```python
from build123d import *

# Parameters (mm, degrees)
BOSS_EXTRUDE1_DEPTH              = 12.7
SKETCH2_R                        = 19.0754
CUT_EXTRUDE2_DEPTH               = 214.127417875
F_10_32_TAPPED_HOLE2_AT_2_COUNT  = 2
F_10_32_TAPPED_HOLE2_AT_2_PITCH  = 101.6
F_10_32_TAPPED_HOLE2_AT_3_COUNT  = 2
F_10_32_TAPPED_HOLE2_AT_3_PITCH  = 199.581369562
F_10_32_TAPPED_HOLE2_AT_4_COUNT  = 2
F_10_32_TAPPED_HOLE2_AT_4_PITCH  = 257.571569241
F_10_32_TAPPED_HOLE2_AT_5_COUNT  = 2
F_10_32_TAPPED_HOLE2_AT_5_PITCH  = 260.369359036
F_10_32_TAPPED_HOLE2_AT_6_COUNT  = 2
F_10_32_TAPPED_HOLE2_AT_6_PITCH  = 236.729200842
F_10_32_TAPPED_HOLE2_AT_7_COUNT  = 2
F_10_32_TAPPED_HOLE2_AT_7_PITCH  = 125.046561074
F_10_32_TAPPED_HOLE2_AT_8_COUNT  = 2
F_10_32_TAPPED_HOLE2_AT_8_PITCH  = 191.941079739
F_1_4_28_TAPPED_HOLE1_AT_2_COUNT = 2
F_1_4_28_TAPPED_HOLE1_AT_2_PITCH = 118.029744238
F_1_4_28_TAPPED_HOLE1_AT_3_COUNT = 2
F_1_4_28_TAPPED_HOLE1_AT_3_PITCH = 162.987319215


with BuildPart() as part:
    # Sketch1 → Boss-Extrude1 (new body)
    with BuildSketch(Plane.XY):
        Polygon((-130.175, -168.275), (130.175, -168.275), (130.175, 60.325), (60.325, 130.175), (-60.325, 130.175), (-130.175, 60.325), align=None)
    extrude(amount=BOSS_EXTRUDE1_DEPTH)

    # Sketch2 → Cut-Extrude2 (cut, through all)
    with BuildSketch(Plane.XY):
        with Locations((0, -57.15)):
            Circle(SKETCH2_R)
    extrude(amount=CUT_EXTRUDE2_DEPTH, mode=Mode.SUBTRACT)

    # Sketch5 → #10-32 Tapped Hole2 (revolve, cut)
    with BuildSketch(Plane(origin=(50.8, 115.8875, 0), x_dir=(0, 1, 0), z_dir=(1, 0, 0))):
        Polygon((0, 0), (0, 12.7), (3.048, 12.7), (2.0193, 11.6713), (2.0193, 1.0287), (3.048, 0), align=None)
    f_10_32_tapped_hole2 = revolve(axis=Axis((50.8, 115.8875, -6.35), (0, 0, 1)), mode=Mode.SUBTRACT)

    # #10-32 Tapped Hole2 at 2: #10-32 Tapped Hole2 ×2
    with Locations(*[(-i * F_10_32_TAPPED_HOLE2_AT_2_PITCH, 0, 0) for i in range(1, F_10_32_TAPPED_HOLE2_AT_2_COUNT)]):
        add(f_10_32_tapped_hole2, mode=Mode.SUBTRACT)

    # #10-32 Tapped Hole2 at 3: #10-32 Tapped Hole2 ×2
    with Locations(*[Vector(-0.8511576023985749, -0.5249102169696354, 0) * (i * F_10_32_TAPPED_HOLE2_AT_3_PITCH) for i in range(1, F_10_32_TAPPED_HOLE2_AT_3_COUNT)]):
        add(f_10_32_tapped_hole2, mode=Mode.SUBTRACT)

    # #10-32 Tapped Hole2 at 4: #10-32 Tapped Hole2 ×2
    with Locations(*[Vector(-0.5547001962252293, -0.8320502943378437, 0) * (i * F_10_32_TAPPED_HOLE2_AT_4_PITCH) for i in range(1, F_10_32_TAPPED_HOLE2_AT_4_COUNT)]):
        add(f_10_32_tapped_hole2, mode=Mode.SUBTRACT)

    # #10-32 Tapped Hole2 at 5: #10-32 Tapped Hole2 ×2
    with Locations(*[Vector(-0.26827273477386476, -0.963343002142514, 0) * (i * F_10_32_TAPPED_HOLE2_AT_5_PITCH) for i in range(1, F_10_32_TAPPED_HOLE2_AT_5_COUNT)]):
        add(f_10_32_tapped_hole2, mode=Mode.SUBTRACT)

    # #10-32 Tapped Hole2 at 6: #10-32 Tapped Hole2 ×2
    with Locations(*[Vector(0.04023584739915886, -0.9991902104124478, 0) * (i * F_10_32_TAPPED_HOLE2_AT_6_PITCH) for i in range(1, F_10_32_TAPPED_HOLE2_AT_6_COUNT)]):
        add(f_10_32_tapped_hole2, mode=Mode.SUBTRACT)

    # #10-32 Tapped Hole2 at 7: #10-32 Tapped Hole2 ×2
    with Locations(*[Vector(0.5459982218929023, -0.8377863341507721, 0) * (i * F_10_32_TAPPED_HOLE2_AT_7_PITCH) for i in range(1, F_10_32_TAPPED_HOLE2_AT_7_COUNT)]):
        add(f_10_32_tapped_hole2, mode=Mode.SUBTRACT)

    # #10-32 Tapped Hole2 at 8: #10-32 Tapped Hole2 ×2
    with Locations(*[Vector(0.35570915873202924, -0.9345967014676182, 0) * (i * F_10_32_TAPPED_HOLE2_AT_8_PITCH) for i in range(1, F_10_32_TAPPED_HOLE2_AT_8_COUNT)]):
        add(f_10_32_tapped_hole2, mode=Mode.SUBTRACT)

    # Sketch7 → 1/4-28 Tapped Hole1 (revolve, cut)
    with BuildSketch(Plane(origin=(105.41, -57.15, 0), x_dir=(0, 1, 0), z_dir=(1, 0, 0))):
        Polygon((0, 0), (0, 12.7), (3.81, 12.7), (2.7051, 11.5951), (2.7051, 1.1049), (3.81, 0), align=None)
    f_1_4_28_tapped_hole1 = revolve(axis=Axis((105.41, -57.15, -6.35), (0, 0, 1)), mode=Mode.SUBTRACT)

    # 1/4-28 Tapped Hole1 at 2: 1/4-28 Tapped Hole1 ×2
    with Locations(*[Vector(-0.09683999633944815, 0.9952999623776622, 0) * (i * F_1_4_28_TAPPED_HOLE1_AT_2_PITCH) for i in range(1, F_1_4_28_TAPPED_HOLE1_AT_2_COUNT)]):
        add(f_1_4_28_tapped_hole1, mode=Mode.SUBTRACT)

    # 1/4-28 Tapped Hole1 at 3: 1/4-28 Tapped Hole1 ×2
    with Locations(*[Vector(-0.35453678407740086, 0.9350420678964421, 0) * (i * F_1_4_28_TAPPED_HOLE1_AT_3_PITCH) for i in range(1, F_1_4_28_TAPPED_HOLE1_AT_3_COUNT)]):
        add(f_1_4_28_tapped_hole1, mode=Mode.SUBTRACT)


solid = part.part
```
Input: part model. Units: mm. Frame: model coordinates. Coordinates: 2 decimals unless noted, no trailing zeros. Loops run counter-clockwise (first coordinate to the right, second up) from the corner with the lowest first, then second, coordinate; pieces in that order, holes last. Notation, with made-up numbers: M -25.75,65.5 L 17.25,65.5 A14 ccw 17.25,92.5 Z; hole C 62.25,52.25 d8. An arc over 180 degrees is marked long. Answer in a Markdown table with one row per item.
1. First-contact query: pin 1 (5.5 mm diameter, centred on x = 119.08, y = 11.13, fed in from +Z); pin 2 (1 mm diameter, centred on x = 95, y = -130, fed in from -Z); pin 3 (2.5 mm diameter, centred on x = 50.8, y = 115.89, fed in from +Z); pin 4 (7 mm diameter, centred on x = 47.625, y = 95.25, fed in from -Z). Flat tips, straight axial feed; report the tip coordinate or a pass-through.
Response:
| item | result |
|---|---|
| pin 1 | stops at z = 12.41 |
| pin 2 | stops at z = 0 |
| pin 3 | passes through |
| pin 4 | stops at z = 0.31 |
2. Section A-A, the plane x = 0. Output: boundary loops of the cut face in (y, z) (3 decimals).
Response:
| item | result |
|---|---|
| outline | M -168.275,0 L -76.225,0 L -76.225,12.7 L -168.275,12.7 Z; M -38.075,0 L 130.175,0 L 130.175,12.7 L -38.075,12.7 Z |
3. Material intervals for line 1 (Y direction, x = 47.5, z = 9.5) (3 decimals); line 2 (X direction, y = 12, z = 9.75) (3 decimals); line 3 (Y direction, x = 50.8, z = 9.5) (3 decimals), sorted ascending.
Response:
| item | result |
|---|---|
| line 1 | y = -168.275 to 92.548, 97.952 to 130.175 |
| line 2 | x = -130.175 to -120.895, -117.255 to 117.255, 120.895 to 130.175 |
| line 3 | y = -168.275 to 113.868, 117.907 to 130.175 |
4. Draft query along Y for faces 1 (the flat face through (95.7, 94.8, 6.3)), 2 (the flat face through (-2, -17, 0)), 3 (the cylindrical face through (-4.14, -75.77, 6.26)). Return one class per face: pulls with the +Y half, pulls with the -Y half, needs draft (parallel to the pull), parting line crosses it, or undercut.
Response:
| item | result |
|---|---|
| face 1 | pulls with the +Y half |
| face 2 | needs draft |
| face 3 | undercut |
5. Section D-D, the plane x = -78.5. Output: boundary loops of the cut face in (y, z) (3 decimals), then the cut area to 3 significant figures.
Response:
| item | result |
|---|---|
| outline | M -168.275,0 L 112,0 L 112,12.7 L -168.275,12.7 Z |
| area | 3,560 mm2 |
6. Section C-C, the plane y = 85.5. Output: boundary loops of the cut face in (x, z), then the cut area to 3 significant figures.
Response:
| item | result |
|---|---|
| outline | M -105,0 L 105,0 L 105,12.7 L -105,12.7 Z |
| area | 2,670 mm2 |
7. Section B-B, the plane z = 7.75. Count the separate pieces of the cut face and the enclosed holes in it, then the cut area to 3 significant figures.
Response:
| item | result |
|---|---|
| separate pieces | 1 |
| enclosed holes | 12 |
| area | 71,500 mm2 |
